Can you work these out from the model? Positions are in its coordinate system, mm. Face numbers are marked on the shaded views. A direction names the side the tool comes from. Coordinates: 2 decimals unless noted, no trailing zeros. Order: outer loops, then holes, each group sorted by start corner. A loop starts at its lowest first (then second) coordinate and runs counter-clockwise, first axis right, second up. Notation, with made-up numbers: (-31.5, 77) -> (-18.5, 77) arc R18 ccw to (-18.5, 89) -> close; hole circle Ø8 at (42, 73.25). An arc over 180 degrees is marked (long way). Answer as a JSON object with one key per item and string values. Group by question number.
(1) For pin 1 (0.6 mm diameter, centred on y = 15.5, z = -0.5, fed in from +X), with a flat end and sliding along its axis, tell me the tip position at first contact or that it passes through.
(2) I want a section at C-C, the plane y = 7.5. List the corners of the cut face in (x, z) for me, plus the area to 3 significant figures.
(3) I want a section at A-A, the plane z = 0. List the corners of the cut face in (x, y) for me, plus the area to 3 significant figures.
(4) I want a section at B-B, the plane x = 13.75. List the corners of the cut face in (y, z) for me.
(5) Which directions (+Z, -Z, +X, -X, +Y, -Y) give clear straight access to the entire face, cutting with the end or side of a thin tool? Please do the marked faces 1 and 2.
(6) I need wall thicknesses on line 1 (Y direction, x = 10, z = -0.55); line 2 (Y direction, x = 12.5, z = -0.05); line 3 (X direction, y = 13.5, z = 0.45). Which ranges of each line are inside material? Lowest first, please.
from build123d import *

# Parameters (mm, degrees)
SWEEP1_PROFILE_R    = 0.65
SKETCH9_R           = 0.35
BOSS_EXTRUDE1_DEPTH = 3


with BuildPart() as part:
    # Sweep1: sweep along a path in Sketch1
    with BuildLine(Plane.XY) as sweep1_path:
        Line((0, 0), (0, 8))
        ThreePointArc((0, 8), (2.050252532, 12.949747468), (7, 15))
        Line((7, 15), (15, 15))
    # Sweep1 profile (on start of the path) → Sweep1 (sweep)
    with BuildSketch(Plane.ZX):
        Circle(SWEEP1_PROFILE_R)
    sweep(path=sweep1_path.line)

    # Sketch9 → Boss-Extrude1 (add)
    with BuildSketch(Plane(origin=(15, 0, 0), x_dir=(0, 0, -1), z_dir=(1, 0, 0))):
        with Locations((0, 15)):
            Circle(SKETCH9_R)
    extrude(amount=BOSS_EXTRUDE1_DEPTH)


solid = part.part
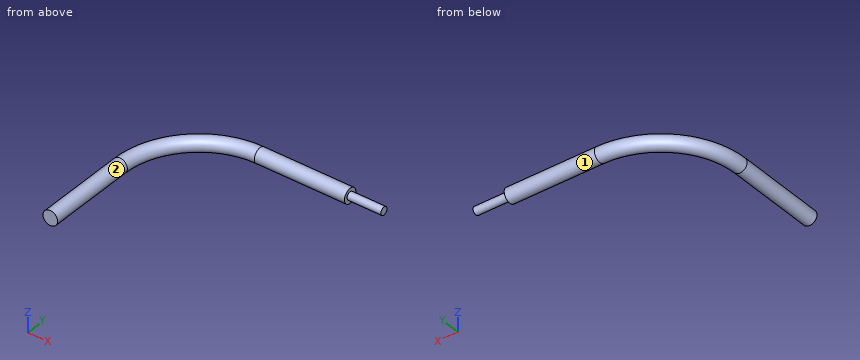
Computed values:
{
 "1": {"pin 1": "stops at x = 15"},
 "2": {"outline": "circle Ø1.3 at (0, 0)", "area": "1.33 mm2"},
 "3": {"outline": "(-0.65, 0) -> (0.65, 0) -> (0.65, 8) arc R6.35 cw to (7, 14.35) -> (15, 14.35) -> (15, 14.65) -> (18, 14.65) -> (18, 15.35) -> (15, 15.35) -> (15, 15.65) -> (7, 15.65) arc R7.65 ccw to (-0.65, 8) -> close", "area": "37.2 mm2"},
 "4": {"outline": "circle Ø1.3 at (15, 0)"},
 "5": {"face 1": "+X", "face 2": "-Y"},
 "6": {"line 1": "y = 14.65 to 15.35", "line 2": "y = 14.35 to 15.65", "line 3": "x = 1.95 to 3.48"}
}
